Autodesk Inventor part; units mm, degrees
ref_plane "Work Plane1" through (-464.1307, 0, 8.7312) normal (-0.1867, 0.9824, 0) x (-0.9824, -0.1867, 0)
ref_plane "YZ Plane" through (0, 0, 0) normal (1, 0, 0) x (0, 1, 0)
ref_plane "XZ Plane" through (0, 0, 0) normal (0, 1, 0) x (-1, 0, 0)
sketch "Sketch1" plane through (0, 0, 0) normal (0, 1, 0) x (-1, 0, 0)
  arc A0 (0, 180.975) -> (146.05, 327.025) centre (146.05, 180.975) ccw
  line L0 (0, 180.975) -> (0, 0)
  line L1 (0, 0) -> (476.25, 0)
  line L2 (476.25, 0) -> (476.25, 327.025)
  line L3 (476.25, 327.025) -> (146.05, 327.025)
  circle A1 centre (301.625, 322.6594) radius 1.5875
  circle A2 centre (441.325, 322.6594) radius 1.5875
  circle A3 centre (371.475, 322.6594) radius 1.5875
  circle A4 centre (231.775, 322.6594) radius 1.5875
  line L4 (450.85, 330.2) -> (450.85, 315.1187) construction
  line L5 (450.85, 330.2) -> (222.25, 330.2) construction
  line L6 (222.25, 315.1187) -> (222.25, 330.2) construction
  line L7 (450.85, 315.1187) -> (222.25, 315.1187) construction
  line L8 (152.5101, 326.2312) -> (152.5101, 327.025) construction
  line L9 (152.5101, 326.2312) -> (177.4637, 326.2312) construction
  line L10 (177.4637, 327.025) -> (177.4637, 326.2312) construction
  line L11 (152.5101, 327.025) -> (177.4637, 327.025) construction
  line L12 (177.4637, 327.025) -> (177.4637, 326.009)
  line L13 (177.4637, 326.009) -> (163.2471, 326.009)
  arc A5 (163.2471, 326.009) -> (146.05, 327.025) centre (146.05, 180.975) ccw
  line L14 (146.05, 327.025) -> (177.4637, 327.025)
  dimension "d0" = 327.025
  dimension "d1" = 330.2
  dimension "d2" = 476.25
  dimension "d3" = 146.05
  dimension "d4" = 180.975
  dimension "d9" = 1.016
extrude "Extrusion1" add sketch "Sketch1" along normal blind 3.175 contours A0 L13 L12 L3 L2 L1 L0
ref_plane "Work Plane1" through (-464.1307, 0, 8.7312) normal (-0.1867, 0.9824, 0) x (-0.9824, -0.1867, 0)
sketch "Sketch2" plane through (-464.1307, 0, 8.7312) normal (-0.1867, 0.9824, 0) x (-0.9824, -0.1867, 0)
  circle A0 centre (7.5406, 223.8375) radius 1.5875
  circle A1 centre (7.5406, 80.9625) radius 1.5875
  circle A2 centre (7.5406, 9.525) radius 1.5875
  circle A3 centre (7.5406, 152.4) radius 1.5875
  circle A4 centre (7.5406, 295.275) radius 1.5875
  line L0 (15.0813, 0) -> (0, 0) construction
  line L1 (15.0813, 0) -> (15.0813, 304.8) construction
  line L2 (0, 304.8) -> (15.0813, 304.8) construction
  line L3 (0, 0) -> (0, 304.8) construction
  point P0 (-455.9729, -8.7312)
extrude "Extrusion2" cut sketch "Sketch2" along normal through all
properties part number "Hopper Bottom" material "Polycarbonate, Clear"
Read the model definition and answer for the solid it produces. Units are mm, in the model's axes. Round coordinates to 2 decimals unless told otherwise and drop trailing zeros. Write each loop counter-clockwise with the first axis right and the second up, starting at its lowest first coordinate (ties: lowest second). Pieces come first, ordered by that corner, then holes.
1. The part is cut by section D-D, the plane z = 265.5. Determine the outline of the cut face in (x, y) (3 decimals), then the cut area to 3 significant figures.
2. The part is cut by section C-C, the plane y = 0.5. State how many separate pieces and enclosed holes the cut face has, then the cut area to 3 significant figures.
3. Straight lines are drawn through the part: L1, parallel to X at y = 0.35, z = 88.5; L2, parallel to Z at x = -144, y = 0.2; L3, parallel to Z at x = -175, y = 0.65. For each, find the intervals that lie inside material, in ascending order.
4. The part is cut by section A-A, the plane x = -259.5. Determine the outline of the cut face in (y, z) (3 decimals).
5. Determine the mould class of faces 1 (the face through (-246.513, 1.565, 74.967)), 2 (the face through (-341, 0, 129)) for opening direction Z: pulls with the +Z half, pulls with the -Z half, needs draft (parallel to the pull), parting line crosses it, or undercut.
6. The part is cut by section B-B, the plane x = -146.05. Determine the outline of the cut face in (y, z) (3 decimals), then the cut area to 3 significant figures.
7. Given pin 1 Ø1.1 at (y, z) = (1, 326.5) entering from +X; pin 2 Ø1.6 at (x, y) = (-168.5, 1) entering from +Z, each flat-ended and moving along its own axis, determine where each tip first touches the part or whether it passes through.
Values:
1. outline: (-476.25, 0) - (-265.156, 0) - (-265.156, 3.175) - (-476.25, 3.175) - close
1. area: 670 mm2
2. separate pieces: 1
2. enclosed holes: 9
2. area: 84,100 mm2
3. L1: x = -476.25 to -472.94, -470.81 to -259.09, -33.01 to 0
3. L2: z = 0 to 34.94
3. L3: z = 0 to 37.82, 324.13 to 326.01
4. outline: (0, 0) - (3.175, 0) - (3.175, 88.998) - (0, 88.998) - close; (0, 272.952) - (3.175, 272.952) - (3.175, 327.025) - (0, 327.025) - close
5. face 1: undercut
5. face 2: needs draft
6. outline: (0, 0) - (3.175, 0) - (3.175, 34.925) - (0, 34.925) - close
6. area: 111 mm2
7. pin 1: stops at x = -163.25
7. pin 2: stops at z = 326.01
